Could you check a few things on this drawing? It's one solid part, dimensions in mm from its lowest x, y, z. A direction names the side the tool comes from. Round coordinates to 2 decimals unless told otherwise and drop trailing zeros. Write each loop counter-clockwise with the first axis right and the second up, starting at its lowest first coordinate (ties: lowest second). Pieces come first, ordered by that corner, then holes. Notation, with made-up numbers: (-35.75, 27) -> (20.25, 27) arc R20 ccw to (20.25, 59) -> close; hole circle Ø2 at (44.25, -2). An arc over 180 degrees is marked (long way). Answer in a Markdown table with one row per item.
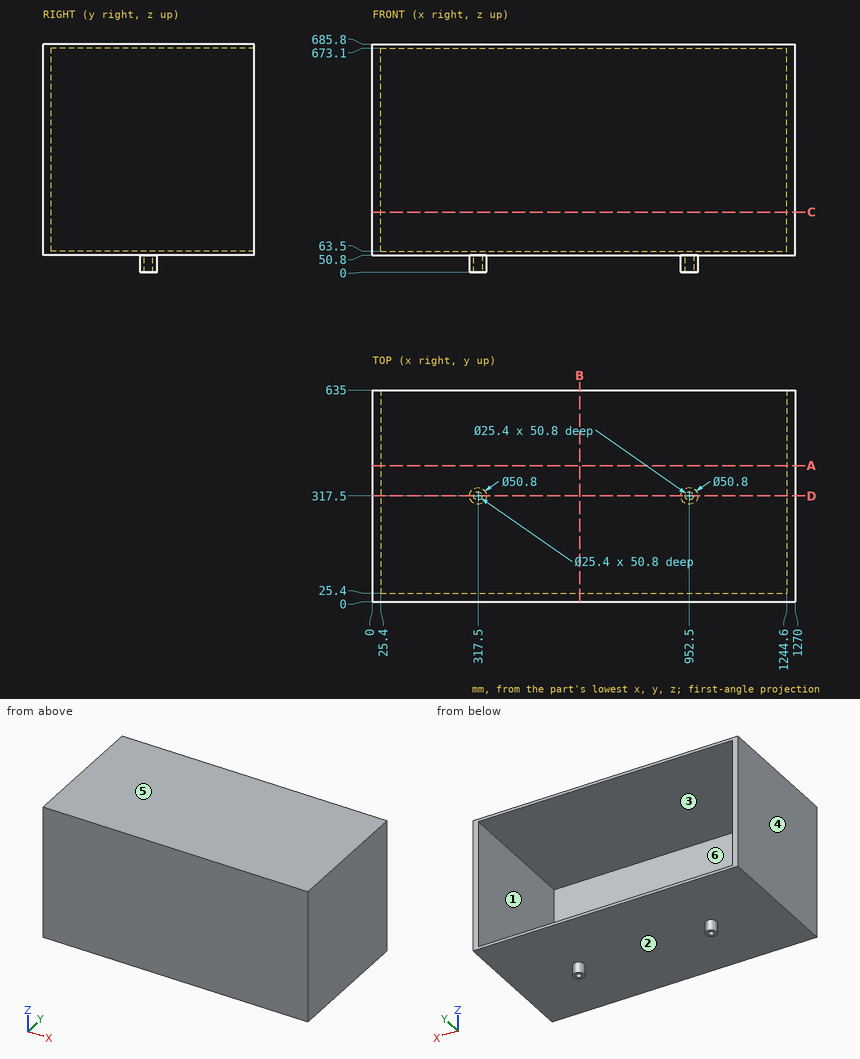
1) I want a section at D-D, the plane y = 317.5. List the corners of the cut face in (x, z) for me.
Response:
| item | result |
|---|---|
| outline | (0, 50.8) -> (292.1, 50.8) -> (292.1, 0) -> (304.8, 0) -> (304.8, 50.8) -> (330.2, 50.8) -> (330.2, 0) -> (342.9, 0) -> (342.9, 50.8) -> (927.1, 50.8) -> (927.1, 0) -> (939.8, 0) -> (939.8, 50.8) -> (965.2, 50.8) -> (965.2, 0) -> (977.9, 0) -> (977.9, 50.8) -> (1270, 50.8) -> (1270, 685.8) -> (0, 685.8) -> close; hole (25.4, 63.5) -> (1244.6, 63.5) -> (1244.6, 673.1) -> (25.4, 673.1) -> close |
2) I need wall thicknesses on line 1 (X direction, y = 317.5, z = 18); line 2 (Y direction, x = 317, z = 33); line 3 (X direction, y = 220.5, z = 231). Which ranges of each line are inside material? Lowest first, please. Write a range as [from, to].
Response:
| item | result |
|---|---|
| line 1 | x = [292.1, 304.8], [330.2, 342.9], [927.1, 939.8], [965.2, 977.9] |
| line 2 | y = [292.1, 304.81], [330.19, 342.9] |
| line 3 | x = [0, 25.4], [1244.6, 1270] |
3) I want a section at A-A, the plane y = 408.5. List the corners of the cut face in (x, z) for me.
Response:
| item | result |
|---|---|
| outline | (0, 50.8) -> (1270, 50.8) -> (1270, 685.8) -> (0, 685.8) -> close; hole (25.4, 63.5) -> (1244.6, 63.5) -> (1244.6, 673.1) -> (25.4, 673.1) -> close |
4) We'd pull the mould along Z, two halves only. Please class the marked faces 1, 2, 3 and 4: +Z half, -Z half, draft (parallel to the pull), parting line (faces both ways), or undercut.
Response:
| item | result |
|---|---|
| face 1 | undercut |
| face 2 | -Z half |
| face 3 | undercut |
| face 4 | draft |
5) For pin 1 (7.5 mm diameter, centred on x = 950.5, y = 311.5, fed in from -Z); pin 2 (1.5 mm diameter, centred on x = 858.5, z = 207, fed in from +Y), each with a flat end and sliding along its axis, tell me the tip position at first contact or that it passes through.
Response:
| item | result |
|---|---|
| pin 1 | stops at z = 50.8 |
| pin 2 | stops at y = 25.4 |
6) I want a section at B-B, the plane x = 623. List the corners of the cut face in (y, z) for me, and give its area (3 significant figures).
Response:
| item | result |
|---|---|
| outline | (0, 50.8) -> (635, 50.8) -> (635, 63.5) -> (25.4, 63.5) -> (25.4, 673.1) -> (635, 673.1) -> (635, 685.8) -> (0, 685.8) -> close |
| area | 31,600 mm^2 |
7) Which directions (+Z, -Z, +X, -X, +Y, -Y) give clear straight access to the entire face, cutting with the end or side of a thin tool? Please do the marked faces 5 and 6.
Response:
| item | result |
|---|---|
| face 5 | +Z, +X, -X, +Y, -Y |
| face 6 | +Y |
8) I want a section at C-C, the plane z = 180.5. List the corners of the cut face in (x, y) for me.
Response:
| item | result |
|---|---|
| outline | (0, 0) -> (1270, 0) -> (1270, 635) -> (1244.6, 635) -> (1244.6, 25.4) -> (25.4, 25.4) -> (25.4, 635) -> (0, 635) -> close |
